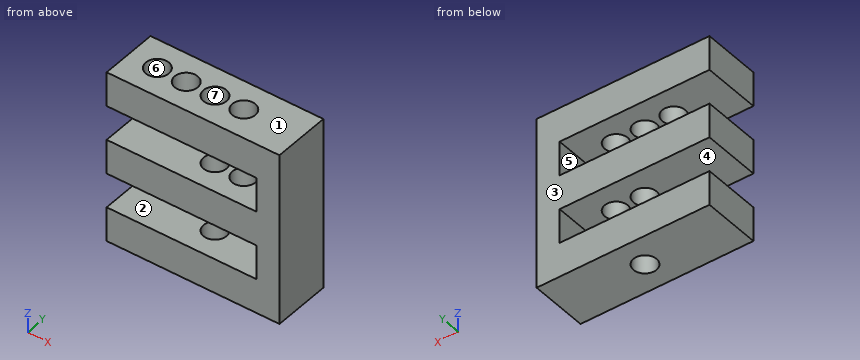
```python
from build123d import *

# Parameters (mm, degrees)
F1_DEPTH = 50
F4_R     = 10
F5_DEPTH = 20
F6_DEPTH = 30
F7_DEPTH = 150.001
F8_DEPTH = 90


with BuildPart() as f1:
    # F0 (on Front) → F1 (new body)
    with BuildSketch(Plane.XZ):
        Polygon((150, 0), (0, 0), (0, -30), (130, -30), (130, -60), (0, -60), (0, -90), (130, -90), (130, -120), (0, -120), (0, -150), (150, -150), align=None)
    extrude(amount=-F1_DEPTH)

    # F4 (on Top) → F5 (cut)
    with BuildSketch(Plane.XY):
        with Locations((25, 25)):
            Circle(F4_R)
    extrude(amount=-F5_DEPTH, mode=Mode.SUBTRACT)

    # F4 (on Top) → F6 (cut, through all)
    with BuildSketch(Plane.XY):
        with Locations((50, 25)):
            Circle(F4_R)
    extrude(amount=-F6_DEPTH, mode=Mode.SUBTRACT)

    # F4 (on Top) → F7 (cut, through all)
    with BuildSketch(Plane.XY):
        with Locations((75, 25)):
            Circle(F4_R)
    extrude(amount=-F7_DEPTH, mode=Mode.SUBTRACT)

    # F4 (on Top) → F8 (cut, through all)
    with BuildSketch(Plane.XY):
        with Locations((100, 25)):
            Circle(F4_R)
    extrude(amount=-F8_DEPTH, mode=Mode.SUBTRACT)


solid = f1.part
```
Input: part model. Units: mm. Frame: model coordinates. Face numbers are marked on the shaded views. A direction names the side the tool comes from. Give positions to 0.01 mm unless a question says otherwise; leave off trailing zeros. Order: outer loops, then holes, each group sorted by start corner. A loop starts at its lowest first (then second) coordinate and runs counter-clockwise, first axis right, second up. Notation, with made-up numbers: (-7.5, 32.5) - (26.5, 32.5) arc R25 ccw to (26.5, 44.5) - close; hole circle Ø10 at (-23, -1.75). An arc over 180 degrees is marked (long way). Put each result on its own line as item: value.
Item 1: Section query D-D, the plane z = -64. Return loops of the section in (x, y), then the cut area to 3 significant figures.
Found:
outline: (0, 0) - (150, 0) - (150, 50) - (0, 50) - close; hole circle Ø20 at (75, 25); hole circle Ø20 at (100, 25)
area: 6,870 mm^2
Item 2: Ray query, L1, parallel to Z at x = 24.5, y = 32; L2, parallel to Z at x = 43, y = 4; L3, parallel to Y at x = 75, z = -80. Return the intervals inside material, ascending. Write a range as from..to.
Found:
L1: z = -150..-120, -90..-60, -30..-20
L2: z = -150..-120, -90..-60, -30..0
L3: y = 0..15, 35..50
Item 3: Section query B-B, the plane x = 50. Return loops of the section in (y, z).
Found:
outline: (0, -150) - (50, -150) - (50, -120) - (0, -120) - close; (0, -90) - (50, -90) - (50, -60) - (0, -60) - close; (0, -30) - (15, -30) - (15, 0) - (0, 0) - close; (35, -30) - (50, -30) - (50, 0) - (35, 0) - close
Item 4: Section query C-C, the plane z = -11. Return loops of the section in (x, y).
Found:
outline: (0, 0) - (150, 0) - (150, 50) - (0, 50) - close; hole circle Ø20 at (25, 25); hole circle Ø20 at (50, 25); hole circle Ø20 at (75, 25); hole circle Ø20 at (100, 25)
Item 5: Section query A-A, the plane x = 75. Return loops of the section in (y, z).
Found:
outline: (0, -150) - (15, -150) - (15, -120) - (0, -120) - close; (0, -90) - (15, -90) - (15, -60) - (0, -60) - close; (0, -30) - (15, -30) - (15, 0) - (0, 0) - close; (35, -150) - (50, -150) - (50, -120) - (35, -120) - close; (35, -90) - (50, -90) - (50, -60) - (35, -60) - close; (35, -30) - (50, -30) - (50, 0) - (35, 0) - close
Item 6: Draft query along Z for the marked faces 1, 2, 3 and 4. Return one class per face: +Z half, -Z half, draft (parallel to the pull), parting line (faces both ways), or undercut.
Found:
face 1: +Z half
face 2: undercut
face 3: draft
face 4: undercut
Item 7: Access query for the marked faces 5, 6 and 7. Directions: +Z, -Z, +X, -X, +Y, -Y. A direction counts if a zero-diameter tool reaches every point of the face in a straight line with its end or side. Return the directions, or none.
Found:
face 5: -X, +Y, -Y
face 6: +Z
face 7: +Z, -Z
Item 8: Contact query for flat-ended pins moving along their axis: pin 1 (2 mm diameter, centred on x = 41.5, y = 32.5, fed in from +Z); pin 2 (10 mm diameter, centred on x = 24, y = 23, fed in from +Z); pin 3 (12 mm diameter, centred on x = 75, y = 25, fed in from -Z); pin 4 (2 mm diameter, centred on y = 23.5, z = -32, fed in from -X). Output: stop coordinate, or through.
Found:
pin 1: stops at z = 0
pin 2: stops at z = -20
pin 3: passes through
pin 4: stops at x = 130
